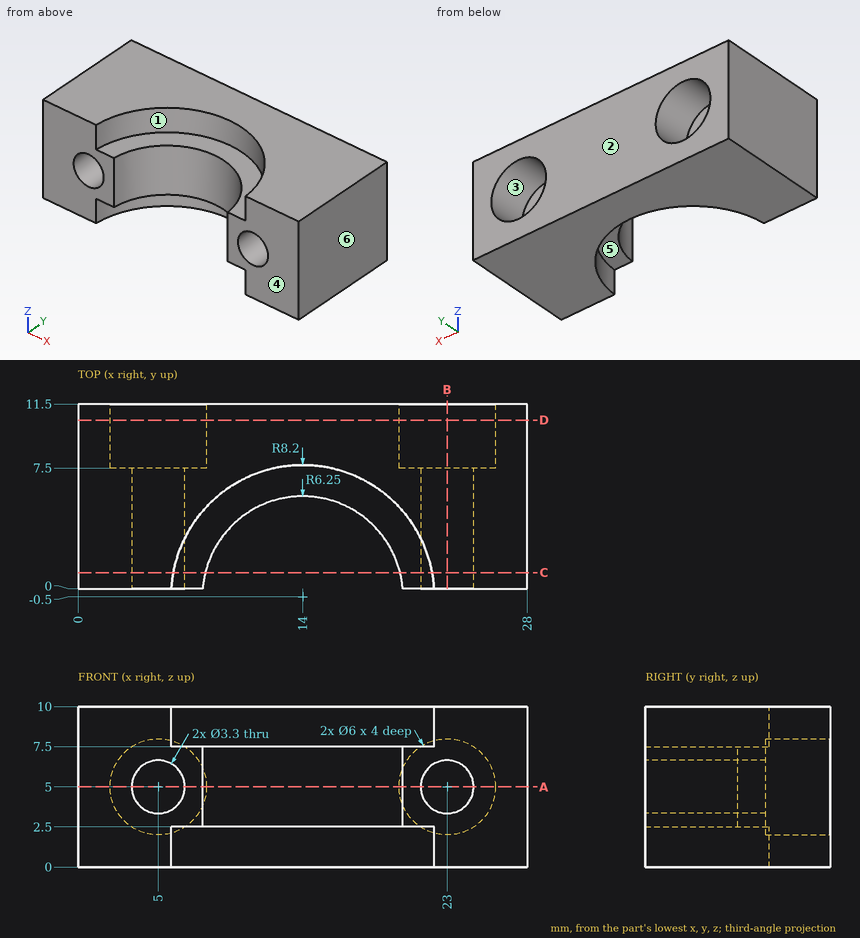
Answer from the drawing. Dimensions are ordinates in mm from the lowest x, y and z of the part. A direction names the side the tool comes from. Coordinates: 2 decimals unless noted, no trailing zeros. Write each loop counter-clockwise with the first axis right and the second up, starting at its lowest first coordinate (ties: lowest second). Pieces come first, ordered by that corner, then holes. Notation, with made-up numbers: (6.25, -13.5) - (15.25, -13.5) arc R20 cw to (15.25, 17.5) - close; hole circle Ø5 at (55, -14.75). An arc over 180 degrees is marked (long way). One line per question, with ' | ' between items.
Q1. Find section B-B, the plane x = 23. Write down the section's boundary in (y, z), plus the area to 4 significant figures.
Result set:
outline: (0, 0) - (11.5, 0) - (11.5, 2) - (7.5, 2) - (7.5, 3.35) - (0, 3.35) - close; (0, 6.65) - (7.5, 6.65) - (7.5, 8) - (11.5, 8) - (11.5, 10) - (0, 10) - close | area: 66.25 mm^2
Q2. Find section C-C, the plane y = 1. Write down the section's boundary in (x, z), plus the area to 3 significant figures.
Result set:
outline: (0, 0) - (5.94, 0) - (5.94, 2.5) - (7.93, 2.5) - (7.93, 7.5) - (5.94, 7.5) - (5.94, 10) - (0, 10) - close; (20.07, 2.5) - (22.06, 2.5) - (22.06, 0) - (28, 0) - (28, 10) - (22.06, 10) - (22.06, 7.5) - (20.07, 7.5) - close; hole circle Ø3.3 at (5, 5); hole circle Ø3.3 at (23, 5) | area: 122 mm^2
Q3. Determine the mould class of the marked faces 4, 5 and 6 for opening direction X: +X half, -X half, draft (parallel to the pull), parting line (faces both ways), or undercut.
Result set:
face 4: draft | face 5: undercut | face 6: +X half
Q4. Find section D-D, the plane y = 10.5. Write down the section's boundary in (x, z), plus the area to 3 significant figures.
Result set:
outline: (0, 0) - (28, 0) - (28, 10) - (0, 10) - close; hole circle Ø6 at (5, 5); hole circle Ø6 at (23, 5) | area: 223 mm^2
Q5. For the marked faces 1, 2 and 3, determine the directions among +Z, -Z, +X, -X, +Y, -Y from which every point of the face is accessible in a straight line to the end or side of a thin tool.
Result set:
face 1: +Z, -Y | face 2: +Z, -Z, +X, -X, +Y | face 3: +Y
Q6. Consider L1, parallel to X at y = 9.5, z = 5; L2, parallel to X at y = 10.5, z = 7.5; L3, parallel to Z at x = 5, y = 9.45. Determine where each line is inside the solid, lowest interval first. Write a range as [from, to].
Result set:
L1: [0, 2], [8, 20], [26, 28] | L2: [0, 3.34], [6.66, 21.34], [24.66, 28] | L3: [0, 2], [8, 10]
Q7. Find section A-A, the plane z = 5. Write down the section's boundary in (x, y).
Result set:
outline: (0, 0) - (3.35, 0) - (3.35, 7.5) - (2, 7.5) - (2, 11.5) - (0, 11.5) - close; (6.65, 0) - (7.77, 0) arc R6.25 cw to (20.23, 0) - (21.35, 0) - (21.35, 7.5) - (20, 7.5) - (20, 11.5) - (8, 11.5) - (8, 7.5) - (6.65, 7.5) - close; (24.65, 0) - (28, 0) - (28, 11.5) - (26, 11.5) - (26, 7.5) - (24.65, 7.5) - close
Q8. Each of these flat-tipped pins is pushed along its axis until it touches: P1, Ø1.8, axis at x = 22.5, z = 4, coming from the +Y side; P2, Ø1.5, axis at x = 11, z = 4.5, coming from the -Y side. Where does it stop, or does it pass through?
Result set:
P1: y = 7.5 | P2: y = 4.5
